The figure shows three views and two pictorial views of one solid part (mm, origin at its lowest corner). Answer the questions. Give positions to 0.01 mm unless a question says otherwise; leave off trailing zeros. Loops run counter-clockwise (first coordinate to the right, second up) from the corner with the lowest first, then second, coordinate; pieces in that order, holes last. Notation, with made-up numbers: (-8, -3.5) - (42, -3.5) arc R23 ccw to (42, 29.5) - close; hole circle Ø5 at (27, -36.5). An arc over 180 degrees is marked (long way). Use a Markdown table: item, result. Add a question column.
Item 1: A cutting plane is placed at A-A (x = 58.5). Determine the outline of the cut face in (y, z).
Item 2: Consider probe 1 along Y at (x, z) = (77, 2.3); probe 2 along X at (y, z) = (36.5, 0.8); probe 3 along Y at (x, z) = (63.5, 1.15). Determine where each line is inside the solid, lowest interval first. Write a range as [from, to].
Item 3: This flat-tipped pin is pushed along its axis until it touches: P1, Ø2.5, axis at x = 77, y = 52, coming from the +Z side. Where does it stop, or does it pass through?
Item 4: A cutting plane is placed at C-C (x = 77). Determine the outline of the cut face in (y, z), plus the area to 3 significant figures.
Item 5: A cutting plane is placed at D-D (z = 1). Give the number of separate pieces and of enclosed holes in the cut face, plus the area to 3 significant figures.
Item 6: A cutting plane is placed at B-B (y = 52). Determine the outline of the cut face in (x, z).
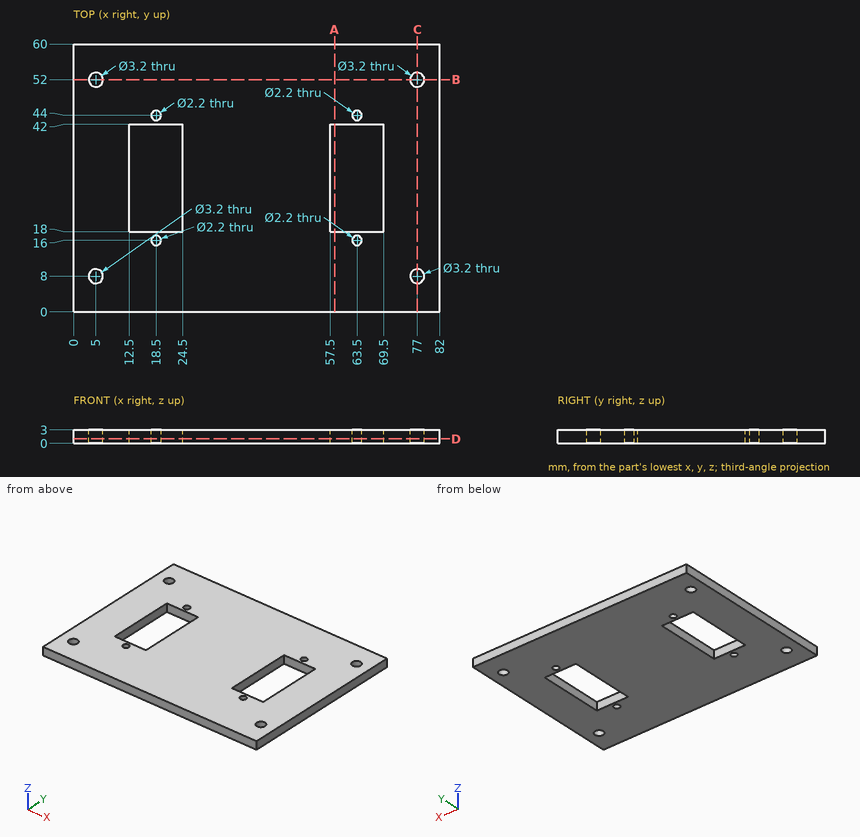
Geometry says:
| question | item | result |
|---|---|---|
| 1 | outline | (0, 0) - (18, 0) - (18, 3) - (0, 3) - close; (42, 0) - (60, 0) - (60, 3) - (42, 3) - close |
| 2 | probe 1 | [0, 6.4], [9.6, 50.4], [53.6, 60] |
| 2 | probe 2 | [0, 12.5], [24.5, 57.5], [69.5, 82] |
| 2 | probe 3 | [0, 14.9], [17.1, 18], [42, 42.9], [45.1, 60] |
| 3 | P1 | through |
| 4 | outline | (0, 0) - (6.4, 0) - (6.4, 3) - (0, 3) - close; (9.6, 0) - (50.4, 0) - (50.4, 3) - (9.6, 3) - close; (53.6, 0) - (60, 0) - (60, 3) - (53.6, 3) - close |
| 4 | area | 161 mm² |
| 5 | separate pieces | 1 |
| 5 | enclosed holes | 10 |
| 5 | area | 4,300 mm² |
| 6 | outline | (0, 0) - (3.4, 0) - (3.4, 3) - (0, 3) - close; (6.6, 0) - (75.4, 0) - (75.4, 3) - (6.6, 3) - close; (78.6, 0) - (82, 0) - (82, 3) - (78.6, 3) - close |
